The listing builds one solid part. Answer for the finished solid, in the listing's coordinates (mm). A direction names the side the tool comes from. Round coordinates to 2 decimals unless told otherwise and drop trailing zeros. Order: outer loops, then holes, each group sorted by start corner. A loop starts at its lowest first (then second) coordinate and runs counter-clockwise, first axis right, second up. Notation, with made-up numbers: (28, -22) - (63, -22) arc R17 cw to (63, -15) - close; hole circle Ø9 at (46, 59.5). An arc over 180 degrees is marked (long way). Write item = value, one per line.
from build123d import *

# Parameters (mm, degrees)
SKETCH1_W           = 181
SKETCH1_H           = 75.57
BOSS_EXTRUDE2_DEPTH = 4.75
SKETCH6_W           = 3
SKETCH6_H           = 10
SKETCH6_W_2         = 10.095812656
SKETCH6_H_2         = 3.003442242
SKETCH6_W_3         = 10
SKETCH6_H_3         = 30
SKETCH6_R           = 1.5
SKETCH6_R_2         = 1.85
SKETCH6_R_3         = 1.75
CUT_EXTRUDE7_DEPTH  = 9


with BuildPart() as part:
    # Sketch1 → Boss-Extrude2 (new body)
    with BuildSketch(Plane.XY):
        Rectangle(SKETCH1_W, SKETCH1_H)
    extrude(amount=BOSS_EXTRUDE2_DEPTH)

    # Sketch6 → Cut-Extrude7 (cut)
    with BuildSketch(Plane.XY.offset(4.75)):
        Polygon((-81.955185068, 35.785), (-81.955183992, 32.802018857), (-71.81277502, 32.798644215), (-71.859372412, 35.785), align=None)
        with Locations((-88, 18.75)):
            Rectangle(SKETCH6_W, SKETCH6_H)
        with Locations((-88, -18.75)):
            Rectangle(SKETCH6_W, SKETCH6_H)
        Polygon((-34.13878131, 35.785), (-34.130786214, 32.798291399), (-24.042968654, 32.781557758), (-24.042968654, 35.785), align=None)
        Polygon((-71.81277502, -32.788413815), (-81.955183992, -32.785039173), (-81.955181828, -35.785039173), (-71.955181828, -35.785031959), align=None)
        Polygon((-33.95518398, -32.801010013), (-33.947153334, -35.800999264), (-23.947156396, -35.808824865), (-23.946905936, -32.804340026), align=None)
        with Locations((87, 9.9)):
            Rectangle(SKETCH6_W, SKETCH6_H)
        with Locations((24.004937674, 34.283278879)):
            Rectangle(SKETCH6_W_2, SKETCH6_H_2)
        Polygon((29.052844002, -32.806257253), (19.053094123, -32.805423656), (19.052844037, -35.805423646), (29.052844002, -35.806257264), align=None)
        with Locations((-8.31156853, 0)):
            Rectangle(SKETCH6_W_3, SKETCH6_H_3)
        with Locations((87, -9.9)):
            Rectangle(SKETCH6_W, SKETCH6_H)
        Polygon((61.466273892, -32.14), (38.055212144, -37.785), (90.5, -37.785), (90.5, -17.2), align=None)
        Polygon((61.46627389, 32.14), (90.5, 18.385572572), (90.5, 37.785), (38.055212144, 37.785), align=None)
        with Locations((-67.23, 30.095)):
            Circle(SKETCH6_R)
        with Locations((-67.23, -30.095)):
            Circle(SKETCH6_R)
        with Locations((70.00651733, -12.753407437)):
            Circle(SKETCH6_R_2)
        with Locations((70.00651733, 12.892480558)):
            Circle(SKETCH6_R_2)
        with Locations((70.00651733, 0)):
            Circle(SKETCH6_R_2)
        with Locations((57.30651733, 12.892480558)):
            Circle(SKETCH6_R_2)
        with Locations((57.30651733, 0)):
            Circle(SKETCH6_R_2)
        with Locations((57.30651733, -12.753407437)):
            Circle(SKETCH6_R_2)
        with Locations((79.833359723, -7.5)):
            Circle(SKETCH6_R_3)
        with Locations((79.833359723, 7.5)):
            Circle(SKETCH6_R_3)
    extrude(amount=-CUT_EXTRUDE7_DEPTH, mode=Mode.SUBTRACT)


solid = part.part
Q1. Section D-D on x = 50 is taken. Determine the outline of the cut face in (y, z), then the cut area to 3 significant figures.
Model answer:
outline = (-34.9, 0) - (34.9, 0) - (34.9, 4.75) - (-34.9, 4.75) - close
area = 332 mm^2
Q2. Section B-B on y = 21 is taken. Determine the outline of the cut face in (x, z), then the cut area to 3 significant figures.
Model answer:
outline = (-90.5, 0) - (-89.5, 0) - (-89.5, 4.75) - (-90.5, 4.75) - close; (-86.5, 0) - (84.98, 0) - (84.98, 4.75) - (-86.5, 4.75) - close
area = 819 mm^2
Q3. Flat-ended cylindrical pins translate along their axes: P1, Ø5, axis at x = -32.5, y = -9, coming from the -Z side; P2, Ø1.5, axis at x = 87.5, z = 2, coming from the -Y side. Find the tip coordinate at first contact, or state that the pin passes through.
Model answer:
P1 = 0
P2 = -19.13
Q4. For faces 4 (the face through (85.5, 10, 2)), 5 (the face through (49.925, -34.923, 2.408)), determine the directions among +Z, -Z, +X, -X, +Y, -Y from which every point of the face is accessible in a straight line to the end or side of a thin tool.
Model answer:
face_4 = +Z, -Z
face_5 = +Z, -Z, +X, -Y
Q5. Section A-A on y = 0 is taken. Determine the outline of the cut face in (x, z).
Model answer:
outline = (-90.5, 0) - (-13.31, 0) - (-13.31, 4.75) - (-90.5, 4.75) - close; (-3.31, 0) - (55.46, 0) - (55.46, 4.75) - (-3.31, 4.75) - close; (59.16, 0) - (68.16, 0) - (68.16, 4.75) - (59.16, 4.75) - close; (71.86, 0) - (90.5, 0) - (90.5, 4.75) - (71.86, 4.75) - close
Q6. Section C-C on z = 2.9 is taken. Count the separate pieces of the cut face and the enclosed holes in it, then the cut area to 3 significant figures.
Model answer:
separate_pieces = 1
enclosed_holes = 21
area = 12,100 mm^2
Q7. Find the intervals of material crossed by line 1 (Y direction, x = -73.5, z = 1.85) (3 decimals); line 2 (X direction, y = -2.5, z = 4); line 3 (X direction, y = 18, z = 1.25), in increasing order. Write a range as from..to.
Model answer:
line_1 = -37.785..-35.785, -32.788..32.799, 35.785..37.785
line_2 = -90.5..-13.31, -3.31..90.5
line_3 = -90.5..-89.5, -86.5..90.5
Q8. Determine the mould class of faces 1 (the face through (-77, -35.785, 2)), 2 (the face through (76.186, -24.565, 2.408)), 3 (the face through (-1, 1, 0)) for opening direction X: released by +X, released by -X, zero draft, split by the parting line, or undercut.
Model answer:
face_1 = undercut
face_2 = released by +X
face_3 = zero draft
